For this review, take the finished solid that the model builds, in its own axes (mm). Round coordinates to 2 decimals unless told otherwise and drop trailing zeros. Loops run counter-clockwise (first coordinate to the right, second up) from the corner with the lowest first, then second, coordinate; pieces in that order, holes last.
1) Take a section at B-B (z = 0). State the section outline as (x, y) points (3 decimals), then the cut area to 4 significant figures.
2) Wall thickness on L1, parallel to X at y = 14.25, z = 0 (3 decimals); L2, parallel to Y at x = -6, z = -30; L3, parallel to X at y = 11, z = -1: over which ranges is each line inside the solid? List them lowest first.
3) Take a section at C-C (x = 0). State the section outline as (y, z) points (3 decimals), then the cut area to 4 significant figures.
4) Take a section at D-D (x = -14). State the section outline as (y, z) points, then the cut area to 3 significant figures.
5) Insertion check: pin 1 (1 mm diameter, centred on x = -21, y = 8, fed in from -Z); pin 2 (3 mm diameter, centred on x = -10.5, y = 2.5, fed in from +Z); pin 3 (1.5 mm diameter, centred on x = 0.5, y = 3.5, fed in from +Z); pin 4 (2 mm diameter, centred on y = 3, z = 27, fed in from -X). Each pin has a flat end and moves straight along its axis. Give the tip position at first contact, or say it passes through.
6) Mouldability with a two-part tool opening along Z and no side actions: class faces 1 (the flat face through (-1.97, 4.93, -9.55)), 2 (the cylindrical face through (7.509, 4.93, 23.846)), 3 (the flat face through (-7.793, 4.93, -7.763)), 4 (the flat face through (-11, 0, 5)) as pulls with the +Z half, pulls with the -Z half, needs draft (parallel to the pull), parting line crosses it, or undercut.
```python
from build123d import *

# Parameters (mm, degrees)
SKETCH1_R           = 25
BOSS_EXTRUDE1_DEPTH = 10
SKETCH2_R           = 34
SKETCH2_R_2         = 2.875
BOSS_EXTRUDE2_DEPTH = 10


with BuildPart() as part:
    # Sketch1 → Boss-Extrude1 (new body)
    with BuildSketch(Plane(origin=(0, 0, 0), x_dir=(1, 0, 0), z_dir=(0, 1, 0))):
        with Locations(Location((0, 0, 0), (0, 0, 270))):
            Circle(SKETCH1_R)
        with BuildLine():
            Line((-1.5, 11), (1.5, 11))
            Line((1.5, 11), (2.425924848, 8.146464793))
            ThreePointArc((2.425924848, 8.146464793), (3.252809175, 7.852976026), (4.045032587, 7.475808409))
            Line((4.045032587, 7.475808409), (6.717514421, 8.838834765))
            Line((6.717514421, 8.838834765), (8.838834765, 6.717514421))
            Line((8.838834765, 6.717514421), (7.475808409, 4.045032587))
            ThreePointArc((7.475808409, 4.045032587), (7.852976026, 3.252809175), (8.146464793, 2.425924848))
            Line((8.146464793, 2.425924848), (11, 1.5))
            Line((11, 1.5), (11, -1.5))
            Line((11, -1.5), (8.146464793, -2.425924848))
            ThreePointArc((8.146464793, -2.425924848), (7.852976026, -3.252809175), (7.475808409, -4.045032587))
            Line((7.475808409, -4.045032587), (8.838834765, -6.717514421))
            Line((8.838834765, -6.717514421), (6.717514421, -8.838834765))
            Line((6.717514421, -8.838834765), (4.045032587, -7.475808409))
            ThreePointArc((4.045032587, -7.475808409), (3.252809175, -7.852976026), (2.425924848, -8.146464793))
            Line((2.425924848, -8.146464793), (1.5, -11))
            Line((1.5, -11), (-1.5, -11))
            Line((-1.5, -11), (-2.425924848, -8.146464793))
            ThreePointArc((-2.425924848, -8.146464793), (-3.252809175, -7.852976026), (-4.045032587, -7.475808409))
            Line((-4.045032587, -7.475808409), (-6.717514421, -8.838834765))
            Line((-6.717514421, -8.838834765), (-8.838834765, -6.717514421))
            Line((-8.838834765, -6.717514421), (-7.475808409, -4.045032587))
            ThreePointArc((-7.475808409, -4.045032587), (-7.852976026, -3.252809175), (-8.146464793, -2.425924848))
            Line((-8.146464793, -2.425924848), (-11, -1.5))
            Line((-11, -1.5), (-11, 1.5))
            Line((-11, 1.5), (-8.146464793, 2.425924848))
            ThreePointArc((-8.146464793, 2.425924848), (-7.852976026, 3.252809175), (-7.475808409, 4.045032587))
            Line((-7.475808409, 4.045032587), (-8.838834765, 6.717514421))
            Line((-8.838834765, 6.717514421), (-6.717514421, 8.838834765))
            Line((-6.717514421, 8.838834765), (-4.045032587, 7.475808409))
            ThreePointArc((-4.045032587, 7.475808409), (-3.252809175, 7.852976026), (-2.425924848, 8.146464793))
            Line((-2.425924848, 8.146464793), (-1.5, 11))
        make_face(mode=Mode.SUBTRACT)
    extrude(amount=BOSS_EXTRUDE1_DEPTH)

    # Sketch2 → Boss-Extrude2 (add)
    with BuildSketch(Plane(origin=(0, 10, 0), x_dir=(1, 0, 0), z_dir=(0, 1, 0))):
        with Locations(Location((0, 0, 0), (0, 0, 270))):
            Circle(SKETCH2_R)
        with Locations(Location((0, 0, 0), (0, 0, 270))):
            Circle(SKETCH2_R_2, mode=Mode.SUBTRACT)
    extrude(amount=BOSS_EXTRUDE2_DEPTH)


solid = part.part
```
Response:
1. outline: (-34, 10) - (-25, 10) - (-25, 0) - (-11, 0) - (-11, 10) - (-2.875, 10) - (-2.875, 20) - (-34, 20) - close; (2.875, 10) - (11, 10) - (11, 0) - (25, 0) - (25, 10) - (34, 10) - (34, 20) - (2.875, 20) - close
1. area: 902.5 mm2
2. L1: x = -34 to -2.875, 2.875 to 34
2. L2: y = 10 to 20
2. L3: x = -33.99 to -2.7, 2.7 to 33.99
3. outline: (0, -25) - (10, -25) - (10, -34) - (20, -34) - (20, -2.875) - (10, -2.875) - (10, -11) - (0, -11) - close; (0, 11) - (10, 11) - (10, 2.875) - (20, 2.875) - (20, 34) - (10, 34) - (10, 25) - (0, 25) - close
3. area: 902.5 mm2
4. outline: (0, -20.71) - (10, -20.71) - (10, -30.98) - (20, -30.98) - (20, 30.98) - (10, 30.98) - (10, 20.71) - (0, 20.71) - close
4. area: 1,030 mm2
5. pin 1: stops at z = -14.31
5. pin 2: stops at z = 23.32
5. pin 3: stops at z = 25
5. pin 4: passes through
6. face 1: undercut
6. face 2: parting line crosses it
6. face 3: undercut
6. face 4: needs draft
